The drawing under review shows one solid part. Ordinate dimensions are in mm from its lowest x, y, z. A direction names the side the tool comes from. Coordinates: 2 decimals unless noted, no trailing zeros. Order: outer loops, then holes, each group sorted by start corner. A loop starts at its lowest first (then second) coordinate and runs counter-clockwise, first axis right, second up. Notation, with made-up numbers: (-25.75, -11.5) -> (0.25, -11.5) arc R11 ccw to (0.25, 0.5) -> close; hole circle Ø8 at (-22, -31). An arc over 180 degrees is marked (long way). Write item = value, one per line.
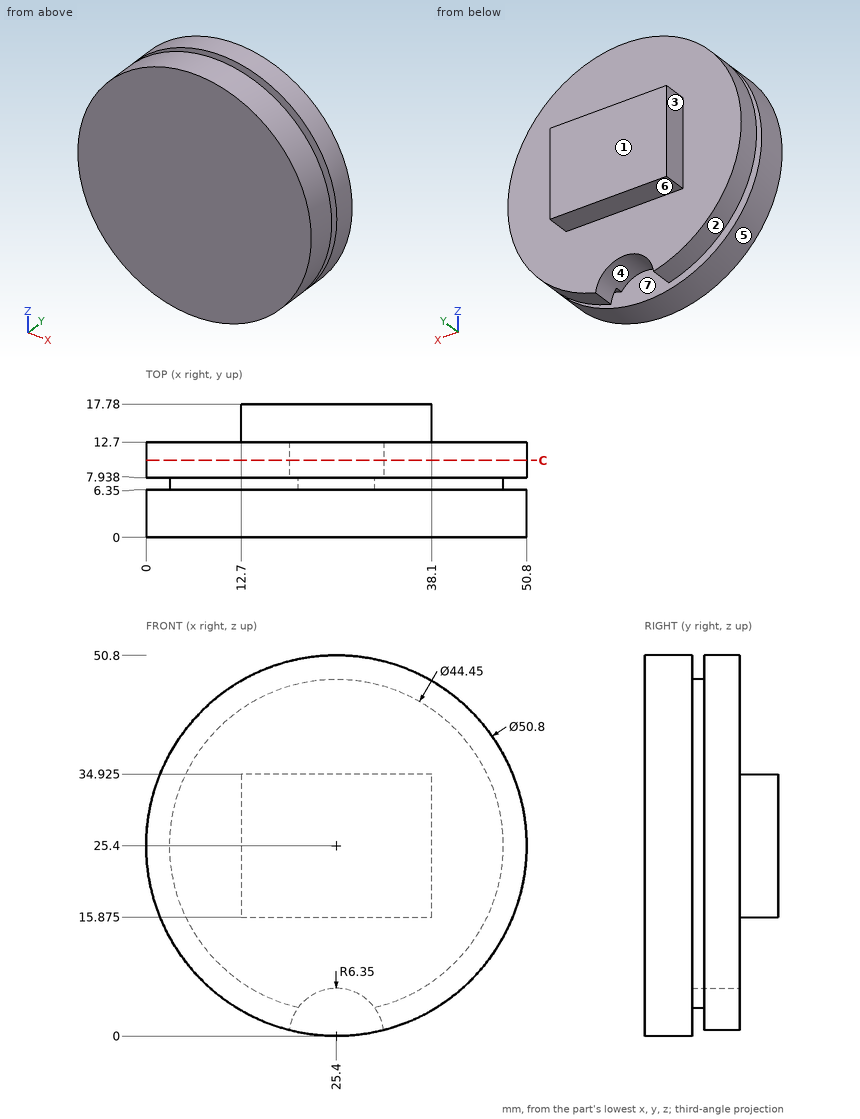
(1) Insertion check: pin 1 (1.5 mm diameter, centred on x = 26.5, y = 15.5, fed in from -Z) (1 decimal); pin 2 (4 mm diameter, centred on y = 4.5, z = 36.5, fed in from +X) (1 decimal); pin 3 (3 mm diameter, centred on x = 23.5, y = 14, fed in from +Z). Each pin has a flat end and moves straight along its axis. Give the tip position at first contact, or say it passes through.
Report:
pin_1 = 15.9
pin_2 = 49.1
pin_3 = 50.77
(2) For the marked faces 5, 6 and 7, list the 3-axis set-ups (+Z, -Z, +X, -X, +Y, -Y) from which the entire face can be reached by the end or side of a thin tool; tool diameter is ignored.
Report:
face_5 = +Y, -Y
face_6 = -Z, +X, -X, +Y
face_7 = none
(3) The part is to be moulded in two halves that separate along X. For the marked faces 1, 2, 3 and 4, say which applies: released by +X, released by -X, zero draft, split by the parting line, or undercut.
Report:
face_1 = zero draft
face_2 = split by the parting line
face_3 = released by -X
face_4 = undercut
(4) For L1, parallel to Y at x = 25, z = 48; L2, parallel to Z at x = 33, y = 13.75 (1 decimal); L3, parallel to X at y = 17, z = 16, list the stretches that pass through material, from the lowest coordinate up.
Report:
L1 = 0 to 6.35, 7.94 to 12.7
L2 = 15.9 to 34.9
L3 = 12.7 to 38.1
(5) We need section C-C (y = 10.25). Write out the cut boundary in (x, z).
Report:
outline = (19.1, 0.79) arc R6.35 cw to (31.7, 0.79) arc R25.4 ccw (long way) to start
